Input: part model. Units: mm. Frame: model coordinates. Face numbers are marked on the shaded views. A direction names the side the tool comes from. Give positions to 0.01 mm unless a question says otherwise; leave off trailing zeros. Write each loop counter-clockwise with the first axis right and the second up, starting at its lowest first coordinate (ties: lowest second). Pieces come first, ordered by that corner, then holes. Notation, with made-up numbers: (7.25, 87) - (41.25, 87) arc R17 ccw to (41.25, 103) - close; hole circle Ø3 at (20.5, 82.5). An arc over 180 degrees is marked (long way). Use a Markdown table: item, result. Add a question column.
1. Section query B-B, the plane y = 937. Return loops of the section in (x, z).
2. Pin query (flat end, axial travel): pin 1 (1.5 mm diameter, centred on y = 335.5, z = -238.5, fed in from -X). Return the tip coordinate at first contact, or that it passes through.
3. Section query A-A, the plane x = -466. Return loops of the section in (y, z), plus the area to 3 significant figures.
4. Mould query, pull axis X, two halves, no side actions, for the marked faces 1, 2, 3 and 4. Classes: released by +X, released by -X, zero draft, split by the parting line, or undercut.
5. Section query C-C, the plane y = 128.5. Return loops of the section in (x, z).
6. Material intervals for probe 1 along X at (y, z) = (56, -505); probe 2 along X at (y, z) = (573, -118); probe 3 along Y at (x, z) = (-739.5, -107), sorted ascending.
7. Set-up query: the marked faces 5, 6 and 7. Return all of +Z, -Z, +X, -X, +Y, -Y with unobstructed straight access to the full face (end or side cutting, diameter ignored); none if empty.
```python
from build123d import *

# Parameters (mm, degrees)
EXTRUDE_1_DEPTH   = 125
EXTRUDE_1_2_DEPTH = 400


with BuildPart() as part:
    # 草图1 → Extrude 1 (new body)
    with BuildSketch(Plane.XY):
        Polygon((-1125, 1125), (-1125, 0), (-1000, 0), (-1000, 1000), (1000, 1000), (1000, 0), (1125, 0), (1125, 1125), align=None)
    extrude(amount=-EXTRUDE_1_DEPTH)

    # 草图2 → Extrude 1 2 (add)
    with BuildSketch(Plane.XZ):
        Polygon((-1000, -125), (-1000, -625), (1000, -625), (1000, -125), (1030, -125), (1030, -655), (-1030, -655), (-1030, -125), align=None)
    extrude(amount=-EXTRUDE_1_2_DEPTH)


solid = part.part
```
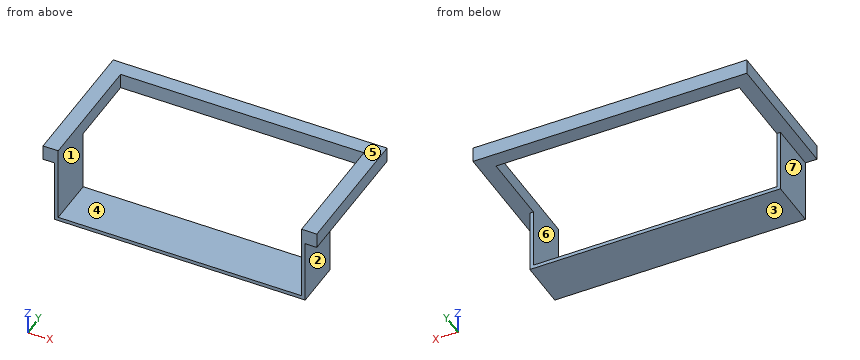
Result sheet:
| question | item | result |
|---|---|---|
| 1 | outline | (-1125, -125) - (-1000, -125) - (-1000, 0) - (-1125, 0) - close; (1000, -125) - (1125, -125) - (1125, 0) - (1000, 0) - close |
| 2 | pin 1 | stops at x = -1030 |
| 3 | outline | (0, -655) - (400, -655) - (400, -625) - (0, -625) - close; (1000, -125) - (1125, -125) - (1125, 0) - (1000, 0) - close |
| 3 | area | 27,600 mm² |
| 4 | face 1 | undercut |
| 4 | face 2 | released by +X |
| 4 | face 3 | zero draft |
| 4 | face 4 | undercut |
| 5 | outline | (-1125, -125) - (-1030, -125) - (-1030, -655) - (1030, -655) - (1030, -125) - (1125, -125) - (1125, 0) - (1000, 0) - (1000, -625) - (-1000, -625) - (-1000, 0) - (-1125, 0) - close |
| 6 | probe 1 | x = -1030 to -1000, 1000 to 1030 |
| 6 | probe 2 | x = -1125 to -1000, 1000 to 1125 |
| 6 | probe 3 | y = 1000 to 1125 |
| 7 | face 5 | +Z, +X, -X, +Y, -Y |
| 7 | face 6 | +Z, -Y |
| 7 | face 7 | -Z, -X, +Y, -Y |
